Answer from the drawing. Dimensions are ordinates in mm from the lowest x, y and z of the part. A direction names the side the tool comes from. Round coordinates to 2 decimals unless told otherwise and drop trailing zeros. Loops run counter-clockwise (first coordinate to the right, second up) from the corner with the lowest first, then second, coordinate; pieces in that order, holes last. Notation, with made-up numbers: M 25.25,67.5 L 29.25,67.5 A12 ccw 29.25,84.5 Z; hole C 84,62 d5. An arc over 180 degrees is marked long. Answer as CSV lines item,"result".
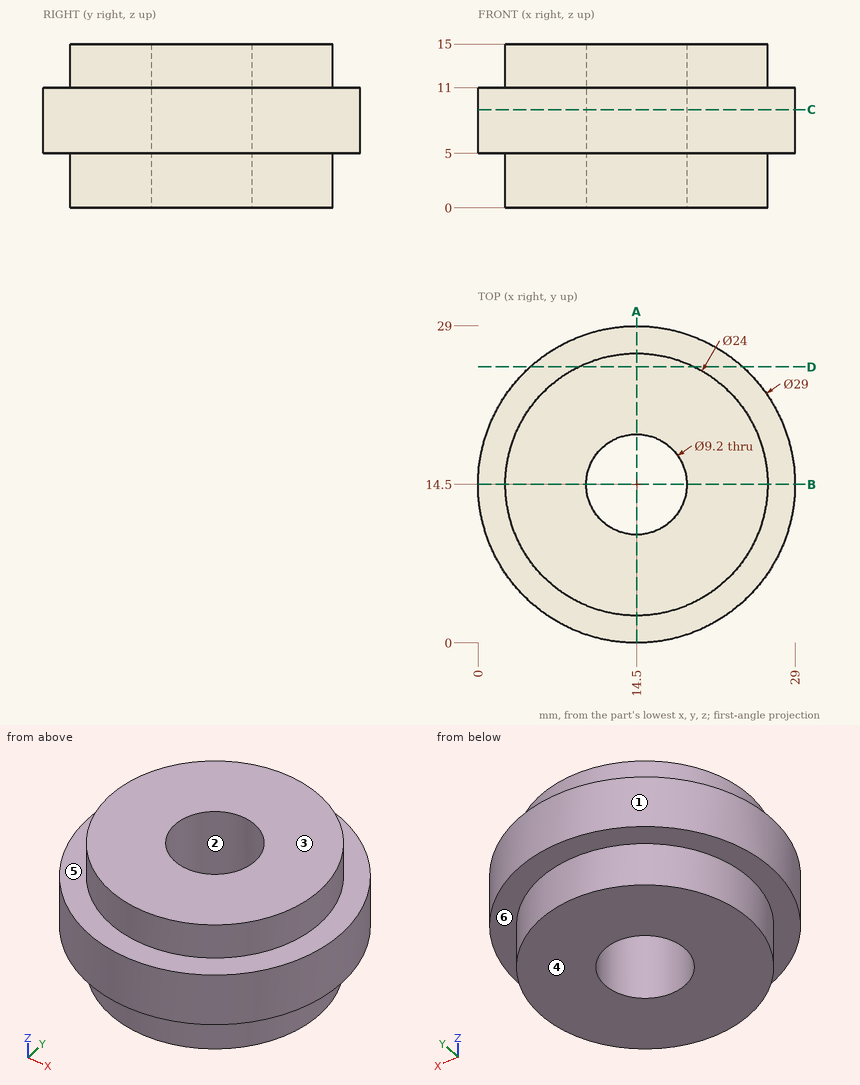
1) Find section D-D, the plane y = 25.25. Give the vertices of the cut face in (x, z).
Evaluation:
outline,"M 4.77,5 L 9.17,5 L 9.17,0 L 19.83,0 L 19.83,5 L 24.23,5 L 24.23,11 L 19.83,11 L 19.83,15 L 9.17,15 L 9.17,11 L 4.77,11 Z"
2) Each of these flat-tipped pins is pushed along its axis until it touches: P1, Ø4, axis at y = 19.5, z = 8.5, coming from the +X side; P2, Ø4, axis at x = 9, z = 9, coming from the +Y side; P3, Ø4, axis at x = 25.5, y = 25, coming from the +Z side. Where does it stop, or does it pass through?
Evaluation:
P1,"stops at x = 28.69"
P2,"stops at y = 28.57"
P3,"stops at z = 11"
3) Find section A-A, the plane x = 14.5. Give the vertices of the cut face in (y, z).
Evaluation:
outline,"M 0,5 L 2.5,5 L 2.5,0 L 9.9,0 L 9.9,15 L 2.5,15 L 2.5,11 L 0,11 Z; M 19.1,0 L 26.5,0 L 26.5,5 L 29,5 L 29,11 L 26.5,11 L 26.5,15 L 19.1,15 Z"
4) Determine the mould class of the marked faces 1, 2 and 3 for opening direction X: released by +X, released by -X, zero draft, split by the parting line, or undercut.
Evaluation:
face 1,"split by the parting line"
face 2,"undercut"
face 3,"zero draft"
5) Find section C-C, the plane z = 9. Give the vertices of the cut face in (x, y), then the cut area to 3 significant figures.
Evaluation:
outline,"C 14.5,14.5 d29; hole C 14.5,14.5 d9.2"
area,"594 mm^2"
6) A tool of negligible diameter and unlimited length cuts with its end or side. For the marked faces 4, 5 and 6, from which of +Z, -Z, +X, -X, +Y, -Y can it reach the whole face along a straight path? Write none if from no direction.
Evaluation:
face 4,"-Z, +X, -X, +Y, -Y"
face 5,"+Z"
face 6,"-Z"
7) Straight lines are drawn through the part: line 1 (X direction, y = 14.5, z = 11.25); line 2 (X direction, y = 14.5, z = 6); line 3 (Z direction, x = 20, y = 3). For each, find the intervals that lie inside material, in ascending order.
Evaluation:
line 1,"x = 2.5 to 9.9, 19.1 to 26.5"
line 2,"x = 0 to 9.9, 19.1 to 29"
line 3,"z = 5 to 11"
